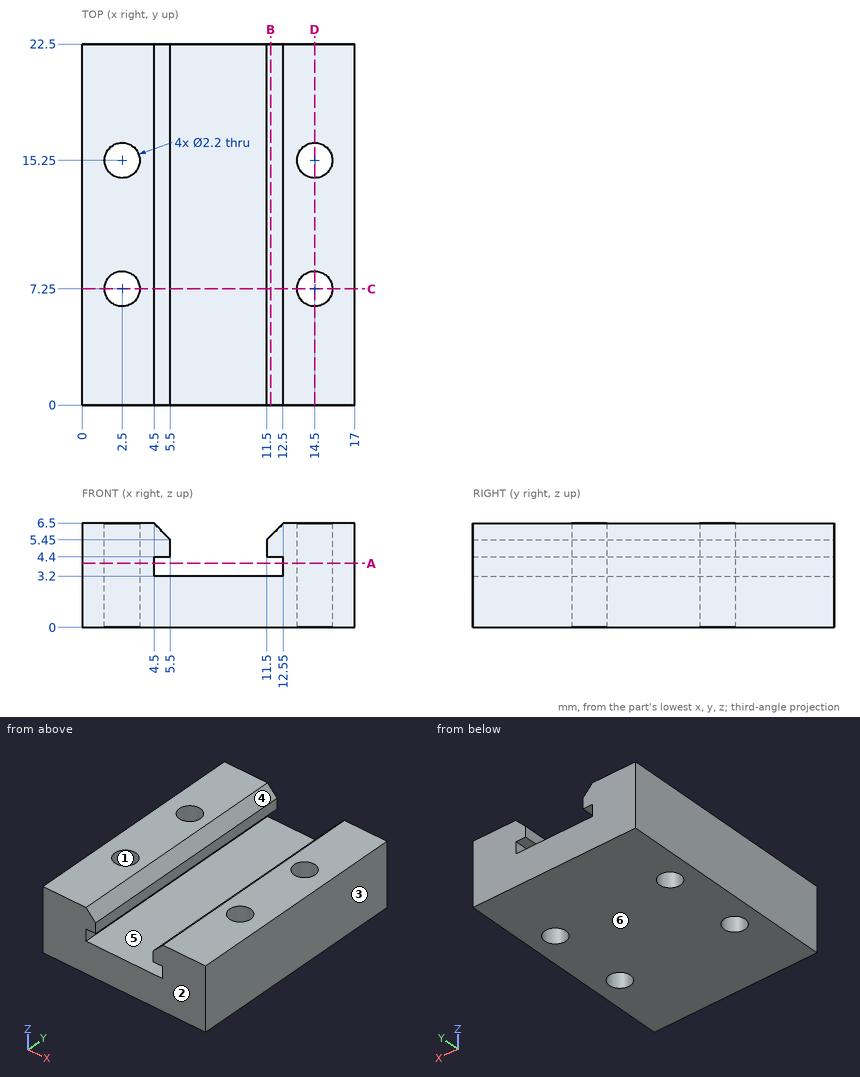
Check sheet for the drawn part. Datum: minimum x, y, z corner. Units: mm. A direction names the side the tool comes from. Round coordinates to 2 decimals unless told otherwise and drop trailing zeros. Write each loop counter-clockwise with the first axis right and the second up, starting at its lowest first coordinate (ties: lowest second). Pieces come first, ordered by that corner, then holes. Notation, with made-up numbers: (-29.5, -8.5) -> (-11.5, -8.5) arc R26 ccw to (-11.5, 6.5) -> close; hole circle Ø11 at (67, 65.25). An arc over 180 degrees is marked (long way). Write each question's results on one line, items separated by ' | '. Start each with the question number.
1. Cross-section at C-C (y = 7.25). Enter the section's corners in (x, z), then the cut area to 3 significant figures.
2. Set-up check for the marked faces 4, 5 and 6: record each of +Z, -Z, +X, -X, +Y, -Y from which the full face is reachable in a straight line by a thin tool's end or side.
3. Draft check along Y on the marked faces 1, 2 and 3. Enter one of: +Y half, -Y half, draft (parallel to the pull), parting line (faces both ways), or undercut.
4. Material ranges on probe 1 along Y at (x, z) = (2.5, 1.75); probe 2 along X at (y, z) = (13.25, 3.5); probe 3 along X at (y, z) = (8, 0.5), recorded low to high. Write a range as from..to.
5. Cross-section at A-A (z = 4). Enter the section's corners in (x, y), then the cut area to 3 significant figures.
6. Cross-section at D-D (x = 14.5). Enter the section's corners in (y, z).
7. Cross-section at B-B (x = 11.75). Enter the section's corners in (y, z), then the cut area to 3 significant figures.
8. Depth check by flat-ended pin: P1, Ø4, axis at x = 9, y = 15, coming from the +Z side. Enter the tip coordinate at first touch or a pass-through.
Solutions:
1) outline: (0, 0) -> (1.4, 0) -> (1.4, 6.5) -> (0, 6.5) -> close; (3.6, 0) -> (13.4, 0) -> (13.4, 6.5) -> (12.55, 6.5) -> (11.5, 5.45) -> (11.5, 4.4) -> (12.5, 4.4) -> (12.5, 3.2) -> (4.5, 3.2) -> (4.5, 4.4) -> (5.5, 4.4) -> (5.5, 5.45) -> (4.5, 6.5) -> (3.6, 6.5) -> close; (15.6, 0) -> (17, 0) -> (17, 6.5) -> (15.6, 6.5) -> close | area: 58.6 mm2
2) face 4: +Z, +Y, -Y | face 5: +Y, -Y | face 6: -Z, +X, -X, +Y, -Y
3) face 1: undercut | face 2: -Y half | face 3: draft
4) probe 1: y = 0..6.15, 8.35..14.15, 16.35..22.5 | probe 2: x = 0..4.5, 12.5..17 | probe 3: x = 0..1.7, 3.3..13.7, 15.3..17
5) outline: (0, 0) -> (4.5, 0) -> (4.5, 22.5) -> (0, 22.5) -> close; (12.5, 0) -> (17, 0) -> (17, 22.5) -> (12.5, 22.5) -> close; hole circle Ø2.2 at (2.5, 7.25); hole circle Ø2.2 at (2.5, 15.25); hole circle Ø2.2 at (14.5, 7.25); hole circle Ø2.2 at (14.5, 15.25) | area: 187 mm2
6) outline: (0, 0) -> (6.15, 0) -> (6.15, 6.5) -> (0, 6.5) -> close; (8.35, 0) -> (14.15, 0) -> (14.15, 6.5) -> (8.35, 6.5) -> close; (16.35, 0) -> (22.5, 0) -> (22.5, 6.5) -> (16.35, 6.5) -> close
7) outline: (0, 0) -> (22.5, 0) -> (22.5, 3.2) -> (0, 3.2) -> close; (0, 4.4) -> (22.5, 4.4) -> (22.5, 5.7) -> (0, 5.7) -> close | area: 101 mm2
8) P1: stops at z = 3.2
